from build123d import *

# Parameters (mm, degrees)
F0_W     = 4
F0_H     = 125
F3_DEPTH = 20
F5_R     = 1


# Not quite as in the source:
# - a fillet or chamfer that OpenCascade refuses, or shapes differently, is made with other operations: its cross-section is extruded or revolved along the edge and cut away or added


with BuildPart() as f1:
    # F0 (on Right) → F1 (revolve)
    with BuildSketch(Plane.YZ):
        with Locations((-2, 0)):
            Rectangle(F0_W, F0_H)
    revolve(axis=Axis((0, 0, 0), (0, 0, -1)))

    # F2 (on face) → F3 (cut)
    with BuildSketch(Plane.XY.offset(62.5)):
        with BuildLine():
            Line((-2.5, 1.6583123952), (-2.5, -1.6583123952))
            ThreePointArc((-2.5, -1.6583123952), (0, -3), (2.5, -1.6583123952))
            Line((2.5, -1.6583123952), (2.5, 1.6583123952))
            ThreePointArc((2.5, 1.6583123952), (0, 3), (-2.5, 1.6583123952))
        make_face()
    extrude(amount=-F3_DEPTH, mode=Mode.SUBTRACT)

    # F4: fillet of radius 3.5 on 1 edges, made by hand

    # F4_s1 → F4_t2 (revolve, cut)
    with BuildSketch(Plane.YZ):
        with BuildLine():
            ThreePointArc((-0.5, 62.5), (-2.9748737342, 61.4748737342), (-4, 59))
            Line((-4, 59), (-4, 62.5))
            Line((-4, 62.5), (-0.5, 62.5))
        make_face()
    revolve(axis=Axis((0, 0, 62.5), (0, 0, -1)), mode=Mode.SUBTRACT)

    # F5
    f5_edges = [f1.edges().sort_by_distance(p)[0] for p in [
        (0, 4, -62.5),
    ]]
    fillet(f5_edges, radius=F5_R)


solid = f1.part
Geometry: final body of the model. Coordinates: model frame, mm. Give positions to 0.01 mm unless a question says otherwise; leave off trailing zeros. Loops run counter-clockwise (first coordinate to the right, second up) from the corner with the lowest first, then second, coordinate; pieces in that order, holes last. Notation, with made-up numbers: (-26, -19) - (8, -19) arc R36 ccw to (8, 17) - close; hole circle Ø10 at (4, 73). An arc over 180 degrees is marked (long way). One line per question, with ' | ' between items. Start each with the question number.
(1) Contact query for flat-ended pins moving along their axis: pin 1 (1.5 mm diameter, centred on x = -1, y = 1, fed in from +Z); pin 2 (2 mm diameter, centred on y = 1, z = -35, fed in from -X); pin 3 (4 mm diameter, centred on x = -0.5, y = 3, fed in from +Z); pin 4 (2 mm diameter, centred on x = -2, z = 34.5, fed in from -Y). Output: stop coordinate, or through.
(2) Pull-direction query (Y, two-part tool) for faces 1 (the flat face through (2.5, 0, 52)), 2 (the flat face through (0, 0, -62.5)), 3 (the cylindrical face through (3.905, 0.867, -0.407)); classes: released by +Y, released by -Y, zero draft, split by the parting line, or undercut.
(3) Section query A-A on z = 33.5. Return loops of the section in (x, y), then the cut area to 3 significant figures.
(4) Ray query, line 1 (Y direction, x = 0, z = 55.5); line 2 (Z direction, x = 0.5, y = 2.5); line 3 (X direction, y = 2.75, z = 52). Return the intervals inside material, ascending. Write a range as from..to.
The answers:
1) pin 1: z = 42.5 | pin 2: x = -4 | pin 3: z = 61.45 | pin 4: y = -3.87
2) face 1: undercut | face 2: zero draft | face 3: split by the parting line
3) outline: circle Ø8 at (0, 0) | area: 50.3 mm2
4) line 1: -4..-3, 3..4 | line 2: -62.5..42.5 | line 3: -2.9..-1.2, 1.2..2.9
